Model file for the job. Use its own axes, mm. A direction names the side the tool comes from. Coordinates: 2 decimals unless noted, no trailing zeros. Write each loop counter-clockwise with the first axis right and the second up, starting at its lowest first coordinate (ties: lowest second). Pieces come first, ordered by that corner, then holes.
Q1. Pin check, flat tips, straight feed: P1, Ø7.5, axis at x = 12, z = -6.5, coming from the +Y side; P2, Ø2.5, axis at x = 18, z = -2, coming from the +Y side; P3, Ø1.6, axis at x = 2, z = -2, coming from the +Y side; P4, Ø1.5, axis at y = 32.5, z = -14, coming from the -X side. Stop position of each tip, or through.
Q2. Pull direction Z, two halves, no side cores. Call faces 1 (the flat face through (5, 30, -17)), 2 (the flat face through (18, 26.5, -18)), 3 (the flat face through (10, 15, -20)): released by +Z, released by -Z, zero draft, split by the parting line, or undercut.
Q3. Band-saw the part on B-B, the plane z = -2. Write the cut outline in (x, y), plus the area to 3 significant figures.
Q4. Which spindle directions (+Z, -Z, +X, -X, +Y, -Y) get a long thin tool onto all of the face, cutting with end or side? Do faces 4 (the cylindrical face through (12, 38, -10)), 5 (the flat face through (10, 0, -10)). Say none if no direction does.
Q5. Band-saw the part on C-C, the plane y = 31. Write the cut outline in (x, z).
Q6. Band-saw the part on A-A, the plane x = 2. Write the cut outline in (y, z).
Q7. Band-saw the part on D-D, the plane z = -15.5. Write the cut outline in (x, y).
Q8. Drill centre lines: probe 1 along X at (y, z) = (28.5, -18); probe 2 along Y at (x, z) = (7.5, -11); probe 3 along Y at (x, z) = (17.75, -3). Where is each one in solid material? Low to high.
from build123d import *

# Parameters (mm, degrees)
SKETCH1_W           = 20
SKETCH1_H           = 20
BOSS_EXTRUDE1_DEPTH = 30
SKETCH2_R           = 1
CUT_EXTRUDE1_DEPTH  = 3.5
SKETCH3_R           = 7.5
BOSS_EXTRUDE2_DEPTH = 1.5
SKETCH4_R           = 2
BOSS_EXTRUDE3_DEPTH = 13.5


with BuildPart() as part:
    # Sketch1 → Boss-Extrude1 (new body)
    with BuildSketch(Plane(origin=(0, 0, 0), x_dir=(1, 0, 0), z_dir=(0, 1, 0))):
        with Locations((10, 10)):
            Rectangle(SKETCH1_W, SKETCH1_H)
    extrude(amount=BOSS_EXTRUDE1_DEPTH)

    # Sketch2 → Cut-Extrude1 (cut)
    with BuildSketch(Plane(origin=(0, 30, 0), x_dir=(1, 0, 0), z_dir=(0, 1, 0))):
        with Locations(Location((2, 18, 0), (0, 0, 270))):
            Circle(SKETCH2_R)
        with Locations(Location((18, 18, 0), (0, 0, 270))):
            Circle(SKETCH2_R)
        with Locations(Location((18, 2, 0), (0, 0, 270))):
            Circle(SKETCH2_R)
        with Locations(Location((2, 2, 0), (0, 0, 270))):
            Circle(SKETCH2_R)
    extrude(amount=-CUT_EXTRUDE1_DEPTH, mode=Mode.SUBTRACT)

    # Sketch3 → Boss-Extrude2 (add)
    with BuildSketch(Plane(origin=(0, 30, 0), x_dir=(1, 0, 0), z_dir=(0, 1, 0))):
        with Locations(Location((10, 10, 0), (0, 0, 90))):
            Circle(SKETCH3_R)
    extrude(amount=BOSS_EXTRUDE2_DEPTH)

    # Sketch4 → Boss-Extrude3 (add)
    with BuildSketch(Plane(origin=(0, 31.5, 0), x_dir=(1, 0, 0), z_dir=(0, 1, 0))):
        with Locations(Location((10, 10, 0), (0, 0, 270))):
            Circle(SKETCH4_R)
    extrude(amount=BOSS_EXTRUDE3_DEPTH)


solid = part.part
Answer sheet:
1. P1: stops at y = 45
1. P2: stops at y = 30
1. P3: stops at y = 26.5
1. P4: passes through
2. face 1: zero draft
2. face 2: undercut
2. face 3: released by -Z
3. outline: (0, 0) - (20, 0) - (20, 30) - (19, 30) - (19, 26.5) - (17, 26.5) - (17, 30) - (3, 30) - (3, 26.5) - (1, 26.5) - (1, 30) - (0, 30) - close
3. area: 586 mm2
4. face 4: +Y
4. face 5: +Z, -Z, +X, -X, -Y
5. outline: circle Ø15 at (10, -10)
6. outline: (0, -20) - (30, -20) - (30, -19) - (26.5, -19) - (26.5, -17) - (30, -17) - (30, -3) - (26.5, -3) - (26.5, -1) - (30, -1) - (30, 0) - (0, 0) - close
7. outline: (0, 0) - (20, 0) - (20, 30) - (15.1, 30) - (15.1, 31.5) - (4.9, 31.5) - (4.9, 30) - (0, 30) - close
8. probe 1: x = 0 to 1, 3 to 17, 19 to 20
8. probe 2: y = 0 to 31.5
8. probe 3: y = 0 to 30
